from build123d import *

# Parameters (mm, degrees)
F1_DEPTH = 7
F2_R     = 11.025
F3_DEPTH = 25.4
F4_R     = 12.7
F5_SIZE  = 2.54


with BuildPart() as f1:
    # F0 (on Front) → F1 (new body)
    with BuildSketch(Plane.XZ):
        with BuildLine():
            Line((-15, 0), (0, 0))
            Line((0, 0), (0, 15))
            ThreePointArc((0, 15), (-13.079524, 13.293907), (-25.25102, 18.377153))
            Line((-25.25102, 18.377153), (-50, 0))
            Line((-50, 0), (-15, 0))
        make_face()
        with BuildLine():
            Line((0, 15), (0, 0))
            Line((0, 0), (15, 0))
            ThreePointArc((15, 0), (13.293907, 13.079524), (18.377153, 25.25102))
            Line((18.377153, 25.25102), (0, 50))
            Line((0, 50), (0, 15))
        make_face()
        with BuildLine():
            Line((0, -15), (0, 0))
            Line((0, 0), (-15, 0))
            ThreePointArc((-15, 0), (-13.293907, -13.079524), (-18.377153, -25.25102))
            Line((-18.377153, -25.25102), (0, -50))
            Line((0, -50), (0, -15))
        make_face()
        with BuildLine():
            Line((15, 0), (0, 0))
            Line((0, 0), (0, -15))
            ThreePointArc((0, -15), (13.079524, -13.293907), (25.25102, -18.377153))
            Line((25.25102, -18.377153), (50, 0))
            Line((50, 0), (15, 0))
        make_face()
    extrude(amount=F1_DEPTH)

    # F2 (on face) → F3 (cut)
    with BuildSketch(Plane.XZ.offset(7)):
        Circle(F2_R)
    extrude(amount=-F3_DEPTH, mode=Mode.SUBTRACT)

    # F4
    f4_edges = [f1.edges().sort_by_distance(p)[0] for p in [
        (0, -3.5, 15),
        (15, -3.5, 0),
        (0, -3.5, -15),
        (-15, -3.5, 0),
    ]]
    fillet(f4_edges, radius=F4_R)

    # F5
    f5_edges = [f1.edges().sort_by_distance(p)[0] for p in [
        (37.62551, 0, -9.188577),
        (37.62551, -7, -9.188577),
        (9.188577, 0, 37.62551),
        (9.188577, -7, 37.62551),
        (-9.188577, 0, -37.62551),
        (-9.188577, -7, -37.62551),
        (-37.62551, 0, 9.188577),
        (-37.62551, -7, 9.188577),
    ]]
    chamfer(f5_edges, length=F5_SIZE)


solid = f1.part
For this review, take the finished solid that the model builds, in its own axes (mm). A direction names the side the tool comes from. Give positions to 0.01 mm unless a question says otherwise; leave off trailing zeros. Loops run counter-clockwise (first coordinate to the right, second up) from the corner with the lowest first, then second, coordinate; pieces in that order, holes last.
Item 1: Insertion check: pin 1 (1.5 mm diameter, centred on y = -2, z = 28.5, fed in from -X); pin 2 (3.5 mm diameter, centred on x = 33, y = -3.5, fed in from +Z); pin 3 (3 mm diameter, centred on x = -5.5, y = -5, fed in from +Z). Each pin has a flat end and moves straight along its axis. Give the tip position at first contact, or say it passes through.
Item 2: Draft analysis for pull direction X (two halves, no side actions). For faces 4 (the flat face through (36.36, -1.29, -8.57)), 5 (the flat face through (38, -3, 0)), 6 (the cylindrical face through (-20.64, -3.45, 15.54)), 7 (the cylindrical face through (-4.97, -3.55, 16.05)), state which applies: +X half, -X half, draft (parallel to the pull), parting line (faces both ways), or undercut.
Item 3: Take a section at B-B, the plane y = -5.75. State the section outline as (x, z) points (3 decimals), and give its area (3 significant figures).
Item 4: Take a section at C-C, the plane x = -3. State the section outline as (y, z) points, and give its area (3 significant figures).
Item 5: For line 1 along X through (y, z) = (-1.25, 17); line 2 along X through (y, z) = (-0.75, 2); line 3 along Z through (x, y) = (-5.5, -5.5), list the stretches that pass through material, from the lowest coordinate up.
Item 6: Take a section at A-A, the plane z = -4. State the section outline as (x, y) points.
Item 7: Tool access review of faces 1 (the cylindrical face through (-15.54, -3.45, -20.64)), 2 (the flat face through (0, -3, -38)), 3 (the cylindrical face through (20.64, -3.45, -15.54)): name each direction out of +Z, -Z, +X, -X, +Y, -Y from which nothing blocks a thin tool from reaching the whole face with its end or side.
Item 8: Take a section at D-D, the plane x = 20. State the section outline as (y, z) points, and give its area (3 significant figures).
Calculated:
1. pin 1: stops at x = 0
1. pin 2: stops at z = 0
1. pin 3: stops at z = 16.87
2. face 4: +X half
2. face 5: draft
2. face 6: undercut
2. face 7: undercut
3. outline: (-47.836, 0) - (-26.126, 0) arc R12.7 cw to (-13.783, -15.688) arc R25.4 cw to (-17.58, -24.161) - (0, -47.836) - (0, -26.126) arc R12.7 cw to (15.688, -13.783) arc R25.4 cw to (24.161, -17.58) - (47.836, 0) - (26.126, 0) arc R12.7 cw to (13.783, 15.688) arc R25.4 cw to (17.58, 24.161) - (0, 47.836) - (0, 26.126) arc R12.7 cw to (-15.688, 13.783) arc R25.4 cw to (-24.161, 17.58) - close; hole circle Ø22.05 at (0, 0)
3. area: 1,950 mm2
4. outline: (-7, -41.7) - (-4.46, -45.96) - (-2.54, -45.96) - (0, -41.7) - (0, -10.61) - (-7, -10.61) - close; (-7, 10.61) - (0, 10.61) - (0, 17.93) - (-7, 17.93) - close
4. area: 288 mm2
5. line 1: x = -24.94 to -23.28, -3.87 to 14.14
5. line 2: x = -44.3 to -10.84, 10.84 to 19.29
5. line 3: z = -40.85 to -9.56, 9.56 to 15.66
6. outline: (-16.87, -7) - (-10.27, -7) - (-10.27, 0) - (-16.87, 0) - close; (10.27, -7) - (40.35, -7) - (44.61, -4.46) - (44.61, -2.54) - (40.35, 0) - (10.27, 0) - close
7. face 1: -X, +Y, -Y
7. face 2: -Z, +X, +Y, -Y
7. face 3: -Z, +Y, -Y
8. outline: (-7, -15.25) - (0, -15.25) - (0, 1.58) - (-7, 1.58) - close
8. area: 118 mm2
